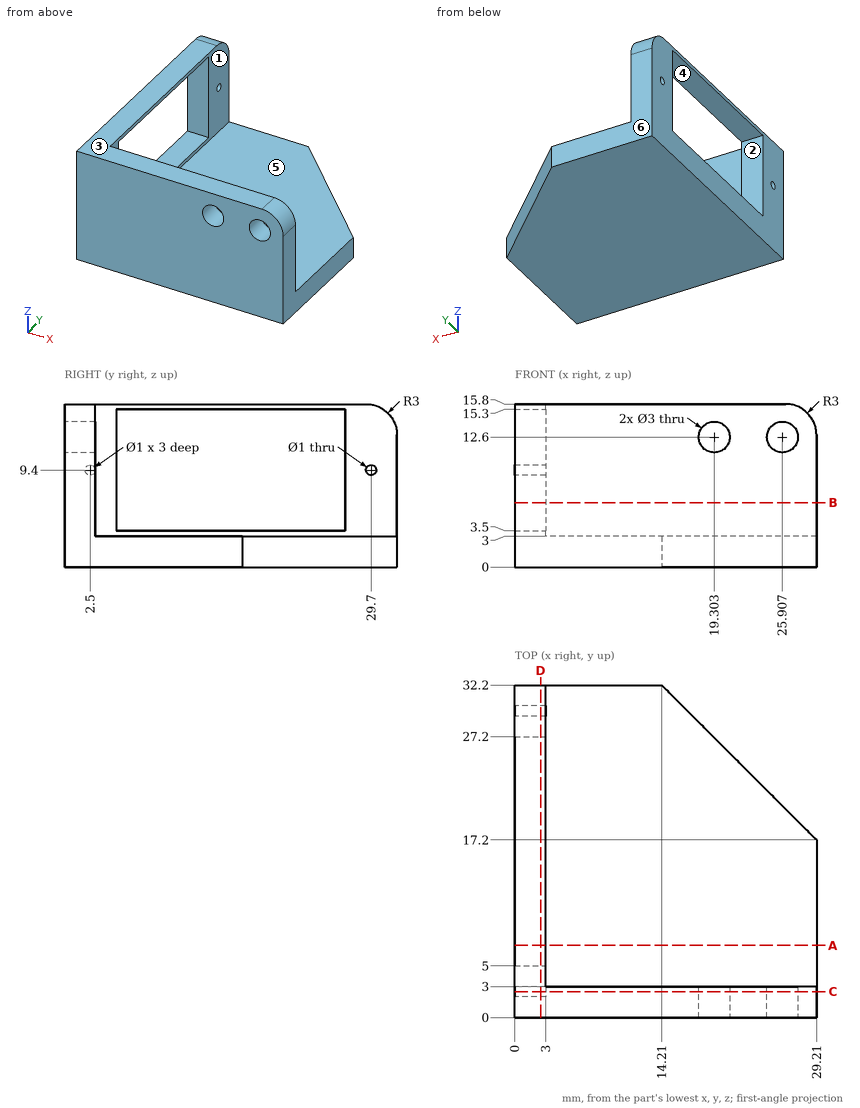
Study the drawing (mm; zero at the part's minimum x, y, z) and answer. A direction names the side the tool comes from. Give positions to 0.01 mm unless a question says otherwise; leave off trailing zeros. Write each loop counter-clockwise with the first axis right and the second up, starting at its lowest first coordinate (ties: lowest second). Pieces come first, ordered by that corner, then holes. Notation, with made-up numbers: (11.5, 47) - (52.5, 47) arc R10 ccw to (52.5, 65) - close; hole circle Ø2 at (-27.5, 13.5). An arc over 180 degrees is marked (long way). One line per question, with ' | ' between items. Start each with the question number.
1. Section D-D, the plane x = 2.5 is taken. Determine the outline of the cut face in (y, z), then the cut area to 3 significant figures.
2. Straight lines are drawn through the part: line 1 (Y direction, x = 1.1, z = 9.4); line 2 (Y direction, x = 21.5, z = 4.25). For each, find the intervals that lie inside material, in ascending order.
3. Given P1, Ø0.9, axis at x = 1.5, z = 11, coming from the -Y side; P2, Ø8, axis at x = 20, y = 23, coming from the +Z side; P3, Ø4, axis at y = 22, z = 3, coming from the +X side; P4, Ø4, axis at y = 6, z = 14, coming from the +X side, each flat-ended and moving along its own axis, determine where each tip first touches the part or whether it passes through.
4. Section C-C, the plane y = 2.5 is taken. Determine the outline of the cut face in (x, z).
5. Determine the mould class of the marked faces 1, 2 and 3 for opening direction Z: +Z half, -Z half, draft (parallel to the pull), parting line (faces both ways), or undercut.
6. Section A-A, the plane y = 7 is taken. Determine the outline of the cut face in (x, z).
7. For the marked faces 4, 5 and 6, determine the directions among +Z, -Z, +X, -X, +Y, -Y from which every point of the face is accessible in a straight line to the end or side of a thin tool.
8. Section B-B, the plane z = 6.25 is taken. Determine the outline of the cut face in (x, y).
Result:
1) outline: (0, 0) - (32.2, 0) - (32.2, 12.8) arc R3 ccw to (29.2, 15.8) - (0, 15.8) - close; hole circle Ø1 at (2.5, 9.4); hole (5, 3.5) - (27.2, 3.5) - (27.2, 15.3) - (5, 15.3) - close; hole circle Ø1 at (29.7, 9.4) | area: 243 mm2
2) line 1: y = 0 to 2, 3 to 5, 27.2 to 29.2, 30.2 to 32.2 | line 2: y = 0 to 3
3) P1: stops at y = 0 | P2: stops at z = 3 | P3: stops at x = 26.41 | P4: stops at x = 3
4) outline: (0, 0) - (29.21, 0) - (29.21, 12.8) arc R3 ccw to (26.21, 15.8) - (0, 15.8) - (0, 9.9) - (3, 9.9) - (3, 8.9) - (0, 8.9) - close; hole circle Ø3 at (19.3, 12.6); hole circle Ø3 at (25.91, 12.6)
5) face 1: draft | face 2: undercut | face 3: +Z half
6) outline: (0, 0) - (29.21, 0) - (29.21, 3) - (3, 3) - (3, 3.5) - (0, 3.5) - close; (0, 15.3) - (3, 15.3) - (3, 15.8) - (0, 15.8) - close
7) face 4: +X, -X | face 5: +Z, +X, +Y | face 6: +Z, -Z, +X, -X, +Y
8) outline: (0, 0) - (29.21, 0) - (29.21, 3) - (3, 3) - (3, 5) - (0, 5) - close; (0, 27.2) - (3, 27.2) - (3, 32.2) - (0, 32.2) - close
